Autodesk Inventor part; units mm, degrees
ref_plane "YZ Plane" through (0, 0, 0) normal (1, 0, 0) x (0, 1, 0)
ref_plane "XZ Plane" through (0, 0, 0) normal (0, 1, 0) x (-1, 0, 0)
ref_plane "XY Plane" through (0, 0, 0) normal (0, 0, 1) x (1, 0, 0)
sketch "Sketch1" plane through (0, 0, 0) normal (0, 0, 1) x (1, 0, 0)
  line L0 (30.9017, 120.8967) -> (30.9017, 145.8967)
  line L1 (30.9017, 145.8967) -> (-30.2983, 145.8967)
  line L2 (-30.2983, 145.8967) -> (-30.2983, 120.8967)
  line L3 (-30.2983, 120.8967) -> (-33.2983, 120.8967)
  line L4 (-33.2983, 120.8967) -> (-33.2983, 89.6967)
  line L5 (-33.2983, 89.6967) -> (-25.2983, 81.6967)
  line L6 (-25.2983, 81.6967) -> (25.9017, 81.6967)
  line L7 (25.9017, 81.6967) -> (33.9017, 89.6967)
  line L8 (33.9017, 89.6967) -> (33.9017, 120.8967)
  line L9 (33.9017, 120.8967) -> (30.9017, 120.8967)
  circle A0 centre (0, 115) radius 20
  circle A1 centre (-23.2983, 138.8967) radius 2.75
  circle A2 centre (23.9017, 91.6967) radius 2.75
  circle A3 centre (23.9017, 138.8967) radius 2.75
  circle A4 centre (-23.2983, 91.6967) radius 2.75
  line L10 (-30.2983, 145.8967) -> (-30.2983, 143.8967)
  line L11 (-30.2983, 143.8967) -> (-28.2983, 143.8967)
  line L12 (-28.2983, 143.8967) -> (28.9017, 143.8967)
  line L13 (28.9017, 143.8967) -> (28.9017, 86.6967)
  line L14 (28.9017, 86.6967) -> (-28.2983, 86.6967)
  line L15 (-28.2983, 86.6967) -> (-28.2983, 143.8967)
  line L16 (0.3017, 86.6967) -> (0.3017, 95.0023)
  line L17 (19.9978, 115.2967) -> (28.9017, 115.2967)
  point P0 (0, 0)
  dimension "d0" = 2
  dimension "d1" = 57.2
extrude "Extrusion1" add sketch "Sketch1" along normal blind 2 contours L12 L13 L17 A0 L16 L14 L15
sketch "Sketch6" plane through (0, 0, 2) normal (0, 0, 1) x (1, 0, 0)
  line L0 (-36.1687, 110.2967) -> (-20.428, 110.2967)
  line L1 (-20.428, 110.2967) -> (-20.428, 120.2967)
  line L2 (-20.428, 120.2967) -> (-36.1687, 120.2967)
  line L3 (-36.1687, 120.2967) -> (-36.1687, 110.2967)
  line L4 (-28.2983, 143.8967) -> (-28.2983, 86.6967)
  line L5 (-36.1687, 110.2967) -> (-20.428, 120.2967) construction
  line L6 (-20.428, 110.2967) -> (-36.1687, 120.2967) construction
  line L7 (-20.428, 120.2967) -> (-50.428, 120.2967)
  line L8 (-50.428, 120.2967) -> (-50.428, 110.2967)
  line L9 (-50.428, 110.2967) -> (-20.428, 110.2967)
  point P0 (0, 0)
  point P1 (-28.2983, 115.2967)
  dimension "d14" = 10
  dimension "d17" = 30
extrude "Extrusion5" add sketch "Sketch6" against normal blind 2
sketch "Sketch7" plane through (0, 0, 2) normal (0, 0, 1) x (1, 0, 0)
  line L0 (-50.428, 110.2967) -> (-50.428, 120.2967)
  line L1 (-50.428, 115.2967) -> (-50.428, 117.2967)
  line L2 (-50.428, 117.2967) -> (-20.428, 117.2967)
  line L3 (-20.428, 117.2967) -> (-20.428, 113.2967)
  line L4 (-20.428, 113.2967) -> (-50.428, 113.2967)
  line L5 (-50.428, 113.2967) -> (-50.428, 115.2967)
  point P0 (0, 0)
  dimension "d18" = 2
  dimension "d19" = 30
  dimension "d20" = 4
extrude "Extrusion6" add sketch "Sketch7" along normal blind 15
sketch "Sketch8" plane through (-50.428, 113.2967, 2) normal (0, -1, 0) x (1, 0, 0)
  circle A0 centre (25, 11) radius 3
  circle A1 centre (5, 11) radius 3
  line L0 (30, 15) -> (30, 7)
  line L1 (30, 15) -> (0, 15)
  line L2 (0, 7) -> (0, 15)
  line L3 (30, 7) -> (0, 7)
  circle A2 centre (25, 11) radius 3
  circle A3 centre (25, 11) radius 1.5
  circle A4 centre (5, 11) radius 1.5
  circle A5 centre (5, 11) radius 3
  circle A6 centre (5, 11) radius 1.5
  point P0 (50.428, -2)
extrude "Extrusion7" add sketch "Sketch8" along normal blind 3 contours A0 | A1
sketch "Sketch9" plane through (-50.428, 113.2967, 2) normal (0, -1, 0) x (1, 0, 0)
  circle A0 centre (25, 11) radius 1.5
  circle A1 centre (5, 11) radius 1.5
  point P0 (50.428, -2)
extrude "Extrusion8" cut sketch "Sketch9" against normal through all
properties part number "stop_rotador_2"
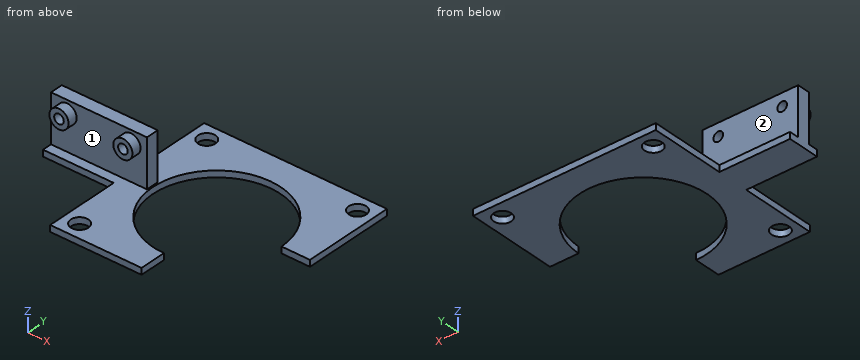
Build history of the part. All positions in model axes, mm. Face numbers are marked on the shaded views. Round coordinates to 2 decimals unless told otherwise and drop trailing zeros. Write each loop counter-clockwise with the first axis right and the second up, starting at its lowest first coordinate (ties: lowest second). Pieces come first, ordered by that corner, then holes. Notation, with made-up numbers: (-19.5, 63) - (-6.5, 63) arc R6 cw to (-6.5, 72) - close; hole circle Ø10 at (43.25, -10). An arc over 180 degrees is marked (long way). Write each question's results on one line, items separated by ' | '. Start each with the question number.
Item 1: Saw through at B-B (y = 130). Write the cut outline in (x, z).
Item 2: Saw through at D-D (x = -41). Write the cut outline in (y, z), and give its area (3 significant figures).
Item 3: Wall check: L1, parallel to Y at x = 0, z = 0.65; L2, parallel to Z at x = -2.5, y = 89.5; L3, parallel to Y at x = -22, z = 15.5. Give the ranges that are in metal, low to high. Write a range as [from, to].
Item 4: Drop flat-ended pins along their axis: P1, Ø1.8, axis at x = -44, z = 13, coming from the -Y side; P2, Ø2, axis at y = 115.5, z = 9, coming from the +X side; P3, Ø10, axis at x = -42, y = 126.5, coming from the +Z side; P4, Ø1, axis at x = -38.5, z = 1, coming from the +Y side. Give the stop position or say it passes through.
Item 5: Saw through at A-A (x = 23). Write the cut outline in (y, z).
Item 6: Saw through at C-C (z = 13). Write the cut outline in (x, y), and give its area (3 significant figures).
Item 7: Mould opens along X. For the marked faces 1 and 2 say: pulls with the +X half, pulls with the -X half, needs draft (parallel to the pull), parting line crosses it, or undercut.
Results are:
1) outline: (-28.3, 0) - (-13.23, 0) - (-13.23, 2) - (-28.3, 2) - close; (13.23, 0) - (28.9, 0) - (28.9, 2) - (13.23, 2) - close
2) outline: (110.3, 0) - (120.3, 0) - (120.3, 2) - (117.3, 2) - (117.3, 17) - (113.3, 17) - (113.3, 2) - (110.3, 2) - close | area: 80.0 mm²
3) L1: y = [86.7, 95], [135, 143.9] | L2: z = [0, 2] | L3: y = [113.3, 117.3]
4) P1: stops at y = 110.3 | P2: stops at x = -20.43 | P3: passes through | P4: stops at y = 120.3
5) outline: (115.3, 0) - (136.3, 0) - (136.3, 2) - (115.3, 2) - close; (141.49, 0) - (143.9, 0) - (143.9, 2) - (141.49, 2) - close
6) outline: (-50.43, 113.3) - (-48.43, 113.3) - (-48.43, 110.3) - (-46.93, 110.3) - (-46.93, 117.3) - (-50.43, 117.3) - close; (-43.93, 110.3) - (-42.43, 110.3) - (-42.43, 113.3) - (-28.43, 113.3) - (-28.43, 110.3) - (-26.93, 110.3) - (-26.93, 117.3) - (-43.93, 117.3) - close; (-23.93, 110.3) - (-22.43, 110.3) - (-22.43, 113.3) - (-20.43, 113.3) - (-20.43, 117.3) - (-23.93, 117.3) - close | area: 114 mm²
7) face 1: undercut | face 2: needs draft
